Check sheet for the drawn part. Datum: minimum x, y, z corner. Units: mm. A direction names the side the tool comes from. Coordinates: 2 decimals unless noted, no trailing zeros. Order: outer loops, then holes, each group sorted by start corner. A loop starts at its lowest first (then second) coordinate and runs counter-clockwise, first axis right, second up. Notation, with made-up numbers: (30, 69.5) -> (38, 69.5) arc R26 cw to (38, 84.5) -> close; hole circle Ø5 at (81, 16.25). An arc over 180 degrees is marked (long way). Write item = value, one per line. Start each with the question number.
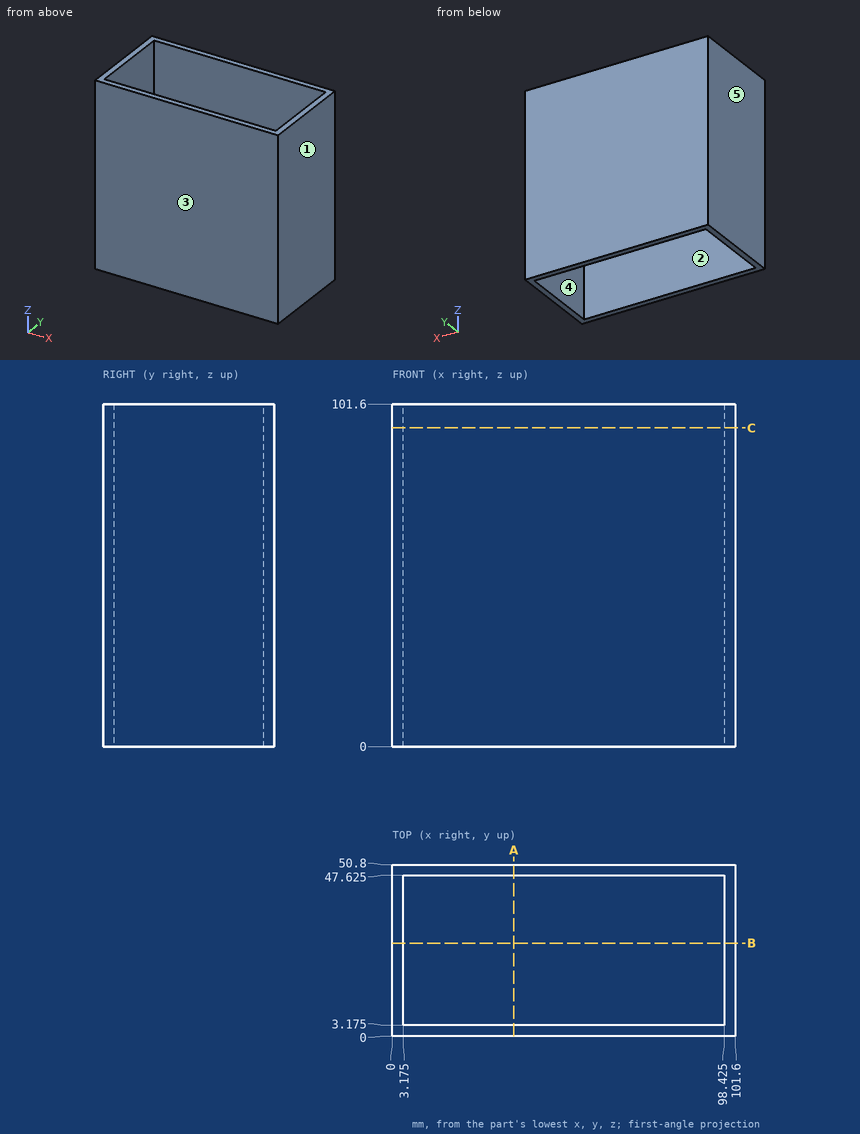
Item 1: Section check A-A (x = 36). Record the boundary of the cut face in (y, z) (3 decimals).
Item 2: Section check C-C (z = 94.5). Record the boundary of the cut face in (x, y) (3 decimals).
Item 3: Tool access check on the marked faces 4 and 5. Record the directions out of +Z, -Z, +X, -X, +Y, -Y that give a thin tool (end or side, any length) a straight path to the whole face; none if there is none.
Item 4: Section check B-B (y = 27.5). Record the boundary of the cut face in (x, z) (3 decimals), then the cut area to 3 significant figures.
Item 5: Thickness scan on line 1 (X direction, y = 43, z = 29.5) (3 decimals); line 2 (Y direction, x = 88, z = 45) (3 decimals). Record the ranges inside material, lowest first.
Item 6: Mould release check, pull along Y, two halves, no side actions. Record for the marked faces 1, 2 and 3: pulls with the +Y half, pulls with the -Y half, needs draft (parallel to the pull), parting line crosses it, or undercut.
Filled sheet:
q1.outline = (0, 0) -> (3.175, 0) -> (3.175, 101.6) -> (0, 101.6) -> close; (47.625, 0) -> (50.8, 0) -> (50.8, 101.6) -> (47.625, 101.6) -> close
q2.outline = (0, 0) -> (101.6, 0) -> (101.6, 50.8) -> (0, 50.8) -> close; hole (3.175, 3.175) -> (98.425, 3.175) -> (98.425, 47.625) -> (3.175, 47.625) -> close
q3.face_4 = +Z, -Z
q3.face_5 = +Z, -Z, -X, +Y, -Y
q4.outline = (0, 0) -> (3.175, 0) -> (3.175, 101.6) -> (0, 101.6) -> close; (98.425, 0) -> (101.6, 0) -> (101.6, 101.6) -> (98.425, 101.6) -> close
q4.area = 645 mm^2
q5.line_1 = 0 to 3.175, 98.425 to 101.6
q5.line_2 = 0 to 3.175, 47.625 to 50.8
q6.face_1 = needs draft
q6.face_2 = undercut
q6.face_3 = pulls with the -Y half
